```python
from build123d import *

# Parameters (mm, degrees)
ESBO_O1_W                = 20
ESBO_O1_H                = 40
ESBO_O1_R                = 3
RESSALTO_EXTRUS_O1_DEPTH = 2.5
FILETE1_R                = 5
ESBO_O2_R                = 2.6
CORTE_EXTRUS_O1_DEPTH    = 6


with BuildPart() as part:
    # Esboço1 → Ressalto-extrusão1 (new, symmetric)
    with BuildSketch(Plane.XY):
        Rectangle(ESBO_O1_W, ESBO_O1_H)
        Circle(ESBO_O1_R, mode=Mode.SUBTRACT)
    extrude(amount=RESSALTO_EXTRUS_O1_DEPTH, both=True)

    # Filete1
    filete1_edges = [part.edges().sort_by_distance(p)[0] for p in [
        (10, -20, 0),
        (-10, -20, 0),
        (-10, 20, 0),
        (10, 20, 0),
    ]]
    fillet(filete1_edges, radius=FILETE1_R)

    # Esboço2 → Corte-extrusão1 (cut)
    with BuildSketch(Plane.XY.offset(2.5)):
        with Locations((0, 15)):
            Circle(ESBO_O2_R)
    corte_extrus_o1 = extrude(amount=-CORTE_EXTRUS_O1_DEPTH, mode=Mode.SUBTRACT)

    # Espelhar1: Corte-extrusão1 across plane
    add(corte_extrus_o1.mirror(Plane.ZX), mode=Mode.SUBTRACT)


solid = part.part
```
Input: part model. Units: mm. Frame: model coordinates. Round coordinates to 2 decimals unless told otherwise and drop trailing zeros. Write each loop counter-clockwise with the first axis right and the second up, starting at its lowest first coordinate (ties: lowest second). Pieces come first, ordered by that corner, then holes. Notation, with made-up numbers: M 22,18.25 L 62,18.25 A17 ccw 62,40.25 Z; hole C 47,-27.5 d8. An arc over 180 degrees is marked long. Write each question's results on one line, items separated by ' | '.
Q1. Section query B-B (z = 0.4). Return loops of the section in (x, y), and give its area (3 significant figures).
Results:
outline: M -10,-15 A5 ccw -5,-20 L 5,-20 A5 ccw 10,-15 L 10,15 A5 ccw 5,20 L -5,20 A5 ccw -10,15 Z; hole C 0,0 d6; hole C 0,-15 d5.2; hole C 0,15 d5.2 | area: 708 mm^2
Q2. Draft query along X for faces 1 (the face through (-0.56, 12.46, 0.04)), 2 (the face through (0, -20, 0)), 3 (the face through (9, 18, 0)), 4 (the face through (-3, 0, 0)). Return one class per face: released by +X, released by -X, zero draft, split by the parting line, or undercut.
Results:
face 1: undercut | face 2: zero draft | face 3: released by +X | face 4: undercut
Q3. Section query A-A (x = 0). Return loops of the section in (y, z), and give its area (3 significant figures).
Results:
outline: M -20,-2.5 L -17.6,-2.5 L -17.6,2.5 L -20,2.5 Z; M -12.4,-2.5 L -3,-2.5 L -3,2.5 L -12.4,2.5 Z; M 3,-2.5 L 12.4,-2.5 L 12.4,2.5 L 3,2.5 Z; M 17.6,-2.5 L 20,-2.5 L 20,2.5 L 17.6,2.5 Z | area: 118 mm^2
Q4. Section query C-C (y = 0). Return loops of the section in (x, z).
Results:
outline: M -10,-2.5 L -3,-2.5 L -3,2.5 L -10,2.5 Z; M 3,-2.5 L 10,-2.5 L 10,2.5 L 3,2.5 Z
Q5. Section query D-D (x = -7.25). Return loops of the section in (y, z).
Results:
outline: M -19.47,-2.5 L 19.47,-2.5 L 19.47,2.5 L -19.47,2.5 Z
Q6. Pin query (flat end, axial travel): P1, Ø3.5, axis at x = 0, y = 0, coming from the +Z side. Return the tip coordinate at first contact, or that it passes through.
Results:
P1: passes through
Q7. Line query: line 1 along Y through (x, z) = (0, -0.6); line 2 along X through (y, z) = (-15, -0.7); line 3 along Y through (x, z) = (-1.5, 1.85). Output: solid intervals per line, ascending.
Results:
line 1: y = -20 to -17.6, -12.4 to -3, 3 to 12.4, 17.6 to 20 | line 2: x = -10 to -2.6, 2.6 to 10 | line 3: y = -20 to -17.12, -12.88 to -2.6, 2.6 to 12.88, 17.12 to 20
